For this review, take the finished solid that the model builds, in its own axes (mm). Round coordinates to 2 decimals unless told otherwise and drop trailing zeros. Write each loop counter-clockwise with the first axis right and the second up, starting at its lowest first coordinate (ties: lowest second). Pieces come first, ordered by that corner, then holes. Notation, with made-up numbers: M -19.5,78 L 32.5,78 A25 ccw 32.5,117 Z; hole C -2.5,55 d1. An arc over 180 degrees is marked long. One line per question, with ' | ' between items.
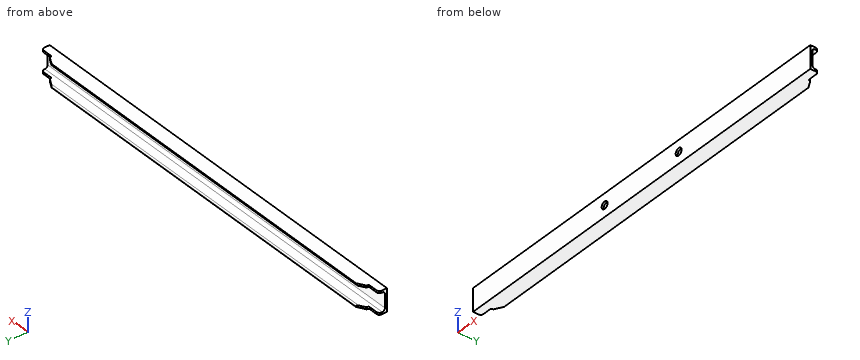
```python
from build123d import *

# Parameters (mm, degrees)
EXTRUDE_1_DEPTH     = 456
SKETCH_2_R          = 8
CUT_EXTRUDE_1_DEPTH = 458.51804336
OTHER_START         = -25
OTHER_1_DEPTH       = 50
CUT_EXTRUDE_2_DEPTH = 461.472800608


# Read off the part's stored shape, not the designer's step: Полость1
with BuildPart() as part:
    # Эскиз1 → Бобышка-Вытянуть1 (new body)
    with BuildSketch(Plane(origin=(0, 0, 0), x_dir=(0, 0, -1), z_dir=(1, 0, 0))):
        with BuildLine():
            Line((25, -39.99), (-25, -39.99))
            Line((-25, -39.99), (-25, -7.99))
            Line((-25, -7.99), (-23.1, -7.99))
            ThreePointArc((-23.1, -7.99), (-21.332233047, -8.722233047), (-20.6, -10.49))
            Line((-20.6, -10.49), (-20.6, -29.59))
            ThreePointArc((-20.6, -29.59), (-18.842640687, -33.832640687), (-14.6, -35.59))
            Line((-14.6, -35.59), (14.6, -35.59))
            ThreePointArc((14.6, -35.59), (18.842640687, -33.832640687), (20.6, -29.59))
            Line((20.6, -29.59), (20.6, -10.49))
            ThreePointArc((20.6, -10.49), (21.332233047, -8.722233047), (23.1, -7.99))
            Line((23.1, -7.99), (25, -7.99))
            Line((25, -7.99), (25, -39.99))
        make_face()
    extrude(amount=-EXTRUDE_1_DEPTH)

    # Эскиз2 → Вырез-Вытянуть1 (cut, through all)
    with BuildSketch(Plane(origin=(0, -35.59, 0), x_dir=(1, 0, 0), z_dir=(0, 1, 0))):
        with Locations(Location((-100, 0, 0), (0, 0, 270))):
            Circle(SKETCH_2_R)
    extrude(amount=-CUT_EXTRUDE_1_DEPTH, mode=Mode.SUBTRACT)

    # Полость1 outline → Полость1 (cut)
    with BuildSketch(Plane.XY.offset(OTHER_START)):
        with BuildLine():
            Line((-428.4, -17.75), (-456, -17.75))
            Line((-456, -17.75), (-456, -28.15))
            ThreePointArc((-456, -28.15), (-454.242640687, -23.907359313), (-450, -22.15))
            Line((-450, -22.15), (-430.9, -22.15))
            ThreePointArc((-430.9, -22.15), (-429.132233047, -21.417766953), (-428.4, -19.65))
            Line((-428.4, -19.65), (-428.4, -17.75))
        make_face()
    extrude(amount=OTHER_1_DEPTH, mode=Mode.SUBTRACT)

    # Эскиз3 → Вырез-Вытянуть2 (cut, through all)
    with BuildSketch(Plane.XY.offset(25)):
        Polygon((-456, -17.75), (-428.4, -17.75), (-411.495184118, -7.99), (-456, -7.99), align=None)
    extrude(amount=-CUT_EXTRUDE_2_DEPTH, mode=Mode.SUBTRACT)

    # Зеркальное отражение1: part across plane


with BuildPart() as part_1:
    add(part.part)
    add(part.part.mirror(Plane(origin=(0, -10.49, 23.1), x_dir=(0, 0, 1), z_dir=(-1, 0, 0))))


solid = part_1.part
```
Item 1: Insertion check: pin 1 Ø3 at (x, z) = (51.5, 3.5) entering from +Y; pin 2 Ø5 at (x, z) = (-441.5, -23.5) entering from +Y; pin 3 Ø0.6 at (y, z) = (-19, 22.5) entering from +X; pin 4 Ø9.5 at (x, z) = (-100, 0) entering from +Y. Each pin has a flat end and moves straight along its axis. Give the tip position at first contact, or say it passes through.
Results:
pin 1: y = -35.59 | pin 2: y = -22.15 | pin 3: x = 428.4 | pin 4: through
Item 2: Take a section at A-A (z = 0). Write out the cut boundary in (x, y), then the cut area to 3 significant figures.
Results:
outline: M -456,-39.99 L -108,-39.99 L -108,-35.59 L -456,-35.59 Z; M -92,-39.99 L 92,-39.99 L 92,-35.59 L -92,-35.59 Z; M 108,-39.99 L 456,-39.99 L 456,-35.59 L 108,-35.59 Z | area: 3,870 mm2
Item 3: To check wall thickness, follow line 1 along X through (y, z) = (-36.7, 0); line 2 along Z through (x, y) = (235, -25.5); line 3 along Z through (x, y) = (100, -36.8). State the ranges of each line that lie inside material, in increasing order. Write a range as from..to.
Results:
line 1: -456..-108, -92..92, 108..456 | line 2: -25..-20.6, 20.6..25 | line 3: -25..-8, 8..25
Item 4: Take a section at B-B (x = -100). Write out the cut boundary in (y, z), then the cut area to 3 significant figures.
Results:
outline: M -39.99,-25 L -7.99,-25 L -7.99,-23.1 A2.5 ccw -10.49,-20.6 L -29.59,-20.6 A6 cw -35.59,-14.6 L -35.59,-8 L -39.99,-8 Z; M -39.99,8 L -35.59,8 L -35.59,14.6 A6 cw -29.59,20.6 L -10.49,20.6 A2.5 ccw -7.99,23.1 L -7.99,25 L -39.99,25 Z | area: 405 mm2
